Build history of the part. All positions in model axes, mm. A direction names the side the tool comes from. Round coordinates to 2 decimals unless told otherwise and drop trailing zeros. Write each loop counter-clockwise with the first axis right and the second up, starting at its lowest first coordinate (ties: lowest second). Pieces come first, ordered by that corner, then holes. Notation, with made-up numbers: (-16, -27.5) -> (6, -27.5) arc R16 ccw to (6, -2.5) -> close; hole circle Ø8 at (56.25, 54). An arc over 180 degrees is marked (long way). Answer as CSV lines item,"result".
Autodesk Inventor part; units mm, degrees
ref_plane "YZ Plane" through (0, 0, 0) normal (1, 0, 0) x (0, 1, 0)
ref_plane "XZ Plane" through (0, 0, 0) normal (0, 1, 0) x (-1, 0, 0)
ref_plane "XY Plane" through (0, 0, 0) normal (0, 0, 1) x (1, 0, 0)
sketch "Skizze1" plane through (0, 0, 0) normal (0, 0, 1) x (1, 0, 0)
  line L0 (0.2, 0) -> (0.5, 0)
  line L1 (0.2, 0) -> (0.5, 0) construction
  line L2 (0.5, 0) -> (1.6547, 2)
  line L3 (1.6547, 2) -> (3.5, 2)
  line L4 (3.5, 2) -> (3.5, 5)
  line L5 (3.5, 5) -> (2.5, 5)
  line L6 (2.5, 5) -> (2.5, 6.5)
  line L7 (2.5, 6.5) -> (3, 6.5)
  line L8 (3, 6.5) -> (3, 21)
  line L9 (3, 21) -> (1, 21)
  line L10 (1, 21) -> (1, 1.9856)
  line L11 (0.2, 0) -> (0.2, 0.6)
  line L12 (0.2, 0.6) -> (1, 1.9856)
  line L13 (0, -4.2) -> (0, 25.2)
  point P0 (0, 0)
  dimension "d4" = 90
  dimension "d6" = 1
  dimension "d7" = 0.2
  dimension "d8" = 0
  dimension "d9" = 0.5
  dimension "d10" = 19
  dimension "d11" = 16
  dimension "d12" = 14.5
  dimension "d13" = 2.5
  dimension "d15" = 21
  dimension "d16" = 0.6
  dimension "d17" = 3.5
  dimension "d18" = 150
  dimension "d19" = 3
revolve "Umdrehung1" add sketch "Skizze1" angle 360 about axis through (0, -10, 0) along (0, 1, 0)
sketch "Skizze2" plane through (0, 2, 0) normal (0, -1, 0) x (1, 0, 0)
  circle A0 centre (0, 0) radius 0.2
  line L0 (3.5412, -1.346) -> (1.5522, -3.4558)
  line L1 (1.5522, -3.4558) -> (-1.346, -3.5412)
  line L2 (-1.346, -3.5412) -> (-3.4558, -1.5522)
  line L3 (-3.4558, -1.5522) -> (-3.5412, 1.346)
  line L4 (-3.5412, 1.346) -> (-1.5522, 3.4558)
  line L5 (-1.5522, 3.4558) -> (1.346, 3.5412)
  line L6 (1.346, 3.5412) -> (3.4558, 1.5522)
  line L7 (3.4558, 1.5522) -> (3.5412, -1.346)
  circle A1 centre (0, 0) radius 1.6547
  dimension "d21" = 7
extrude "Extrusion2" add sketch "Skizze2" against normal up to surface (3 mm away) contours L0 L1 L2 L3 L4 L5 L6 L7
thread "Gewinde1"
chamfer "Fase1" distance 0.5 angle 45 2 edges at (-3, 6.5, 0) (-3, 21, 0)
properties part number "E3D-v6 Volcano Nozzle" material "Messing, weicher Gelbton"
1. Mould opens along X. For faces 4 (the flat face through (2.386, 3.479, 2.561)), 5 (the cylindrical face through (0, 11, -1)), 6 (the flat face through (1, 21, 1)), 7 (the conical face through (-0.093, 0.995, 0.418)) say: +X half, -X half, draft (parallel to the pull), parting line (faces both ways), or undercut.
Results found:
face 4,"+X half"
face 5,"undercut"
face 6,"draft"
face 7,"undercut"
2. Probe line 1 along Z through (x, y) = (0, 15); line 2 along Y through (x, z) = (-1.5, -3); line 3 along Y through (x, z) = (-0.75, 2). List the from-to ranges inside material, lowest first.
Results found:
line 1,"z = -3 to -1, 1 to 3"
line 2,"y = 2 to 5"
line 3,"y = 2 to 21"
3. Cut at D-D, the plane x = 3.25. Write the cut outline in (y, z).
Results found:
outline,"(2, -1.65) -> (5, -1.65) -> (5, 1.75) -> (2, 1.75) -> close"
4. Which spindle directions (+Z, -Z, +X, -X, +Y, -Y) get a long thin tool onto all of the face, cutting with end or side? Do faces 1 (the flat face through (-2, 5, 2)), 2 (the flat face through (-2, 2, -1)), 3 (the flat face through (2.561, 3.479, -2.386)). Say none if no direction does.
Results found:
face 1,"none"
face 2,"-Y"
face 3,"-Z, +X, +Y, -Y"
5. Drop flat-ended pins along their axis: pin 1 Ø3 at (y, z) = (15, 2) entering from +X; pin 2 Ø4 at (y, z) = (12.5, -0.5) entering from -X; pin 3 Ø3 at (x, y) = (2.5, 9) entering from -Z. Give the stop position or say it passes through.
Results found:
pin 1,"stops at x = 2.96"
pin 2,"stops at x = -3"
pin 3,"stops at z = -2.83"
6. Cut at B-B, the plane y = 4.75. Write the cut outline in (x, z), then the cut area to 3 significant figures.
Results found:
outline,"(-3.54, 1.35) -> (-3.46, -1.55) -> (-1.35, -3.54) -> (1.55, -3.46) -> (3.54, -1.35) -> (3.46, 1.55) -> (1.35, 3.54) -> (-1.55, 3.46) -> close; hole circle Ø2 at (0, 0)"
area,"37.5 mm2"
